```python
from build123d import *

# Parameters (mm, degrees)
SKETCH_1_W          = 80
SKETCH_1_H          = 118.5
SKETCH_1_W_2        = 35
SKETCH_1_H_2        = 15
EXTRUDE_1_DEPTH     = 3
CUT_EXTRUDE_2_REACH = 145.008
SKETCH_3_R          = 1.55
CUT_EXTRUDE_3_REACH = 145.008
SKETCH_4_R          = 1.55


with BuildPart() as part:
    # 草图1 → 凸台-拉伸1 (new body)
    with BuildSketch(Plane.XY):
        with Locations((40, 59.25)):
            Rectangle(SKETCH_1_W, SKETCH_1_H)
        with Locations((40, 59.25)):
            Rectangle(SKETCH_1_W_2, SKETCH_1_H_2, mode=Mode.SUBTRACT)
    extrude(amount=EXTRUDE_1_DEPTH)

    # 草图3 → 切除-拉伸2 (cut, up to next)
    with BuildSketch(Plane.XY.offset(3), mode=Mode.PRIVATE) as cut_extrude_2_sk1:
        with Locations((10, 113.5)):
            Circle(SKETCH_3_R)
    cut_extrude_2_tool1 = extrude(cut_extrude_2_sk1.sketch, amount=-CUT_EXTRUDE_2_REACH, mode=Mode.PRIVATE) & part.part
    # 草图3 → 切除-拉伸2 (cut, up to next)
    with BuildSketch(Plane.XY.offset(3), mode=Mode.PRIVATE) as cut_extrude_2_sk2:
        with Locations((70, 113.5)):
            Circle(SKETCH_3_R)
    cut_extrude_2_tool2 = extrude(cut_extrude_2_sk2.sketch, amount=-CUT_EXTRUDE_2_REACH, mode=Mode.PRIVATE) & part.part
    # 草图3 → 切除-拉伸2 (cut, up to next)
    with BuildSketch(Plane.XY.offset(3), mode=Mode.PRIVATE) as cut_extrude_2_sk3:
        with Locations((70, 5)):
            Circle(SKETCH_3_R)
    cut_extrude_2_tool3 = extrude(cut_extrude_2_sk3.sketch, amount=-CUT_EXTRUDE_2_REACH, mode=Mode.PRIVATE) & part.part
    # 草图3 → 切除-拉伸2 (cut, up to next)
    with BuildSketch(Plane.XY.offset(3), mode=Mode.PRIVATE) as cut_extrude_2_sk4:
        with Locations((10, 5)):
            Circle(SKETCH_3_R)
    cut_extrude_2_tool4 = extrude(cut_extrude_2_sk4.sketch, amount=-CUT_EXTRUDE_2_REACH, mode=Mode.PRIVATE) & part.part
    add(cut_extrude_2_tool1.solids().sort_by_distance((10, 113.5, 3))[0], mode=Mode.SUBTRACT)
    add(cut_extrude_2_tool2.solids().sort_by_distance((70, 113.5, 3))[0], mode=Mode.SUBTRACT)
    add(cut_extrude_2_tool3.solids().sort_by_distance((70, 5, 3))[0], mode=Mode.SUBTRACT)
    add(cut_extrude_2_tool4.solids().sort_by_distance((10, 5, 3))[0], mode=Mode.SUBTRACT)

    # 草图4 → 切除-拉伸3 (cut, up to next)
    with BuildSketch(Plane(origin=(0, 0, 0), x_dir=(-1, 0, 0), z_dir=(0, 0, -1)), mode=Mode.PRIVATE) as cut_extrude_3_sk1:
        with Locations((-67, 59.25)):
            Circle(SKETCH_4_R)
    cut_extrude_3_tool1 = extrude(cut_extrude_3_sk1.sketch, amount=-CUT_EXTRUDE_3_REACH, mode=Mode.PRIVATE) & part.part
    # 草图4 → 切除-拉伸3 (cut, up to next)
    with BuildSketch(Plane(origin=(0, 0, 0), x_dir=(-1, 0, 0), z_dir=(0, 0, -1)), mode=Mode.PRIVATE) as cut_extrude_3_sk2:
        with Locations((-13, 59.25)):
            Circle(SKETCH_4_R)
    cut_extrude_3_tool2 = extrude(cut_extrude_3_sk2.sketch, amount=-CUT_EXTRUDE_3_REACH, mode=Mode.PRIVATE) & part.part
    add(cut_extrude_3_tool1.solids().sort_by_distance((67, 59.25, 0))[0], mode=Mode.SUBTRACT)
    add(cut_extrude_3_tool2.solids().sort_by_distance((13, 59.25, 0))[0], mode=Mode.SUBTRACT)


solid = part.part
```
CAD build for the part. Positions are in the model's coordinates, mm. A direction names the side the tool comes from. Round coordinates to 2 decimals unless told otherwise and drop trailing zeros. Write each loop counter-clockwise with the first axis right and the second up, starting at its lowest first coordinate (ties: lowest second). Pieces come first, ordered by that corner, then holes. Notation, with made-up numbers: (20, -9.75) - (50, -9.75) arc R21 cw to (50, -2.75) - close; hole circle Ø2 at (65, -13). An arc over 180 degrees is marked (long way). Write item = value, one per line. Start each with the question number.
Q1. Mould opens along X. For faces 3 (the flat face through (80, 58, 1)), 4 (the flat face through (40, 66.75, 1)), 5 (the flat face through (0, 58, 1)) say: pulls with the +X half, pulls with the -X half, needs draft (parallel to the pull), parting line crosses it, or undercut.
Q2. Band-saw the part on D-D (x = 13). Give the cut face in (y, z).
Q3. Band-saw the part on B-B (z = 1.8). Give the cut face in (x, y).
Q4. Which spindle directions (+Z, -Z, +X, -X, +Y, -Y) get a long thin tool onto all of the face, cutting with end or side? Do faces 1 (the flat face through (39, 0, 1)), 2 (the flat face through (57.5, 59, 1)). Say none if no direction does.
Q5. Band-saw the part on C-C (x = 70). Give the cut face in (y, z).
Q6. Probe L1, parallel to Y at x = 70, z = 0.65; L2, parallel to Y at x = 13, z = 2.15; L3, parallel to Y at x = 27.5, z = 2. List the from-to ranges inside material, lowest first. Write a range as from..to.
Q7. Band-saw the part on A-A (x = 47). Give the cut face in (y, z).
Answers below:
q1.face_3 = pulls with the +X half
q1.face_4 = undercut
q1.face_5 = pulls with the -X half
q2.outline = (0, 0) - (57.7, 0) - (57.7, 3) - (0, 3) - close; (60.8, 0) - (118.5, 0) - (118.5, 3) - (60.8, 3) - close
q3.outline = (0, 0) - (80, 0) - (80, 118.5) - (0, 118.5) - close; hole circle Ø3.1 at (10, 5); hole circle Ø3.1 at (10, 113.5); hole circle Ø3.1 at (13, 59.25); hole (22.5, 51.75) - (57.5, 51.75) - (57.5, 66.75) - (22.5, 66.75) - close; hole circle Ø3.1 at (67, 59.25); hole circle Ø3.1 at (70, 5); hole circle Ø3.1 at (70, 113.5)
q4.face_1 = +Z, -Z, +X, -X, -Y
q4.face_2 = +Z, -Z
q5.outline = (0, 0) - (3.45, 0) - (3.45, 3) - (0, 3) - close; (6.55, 0) - (111.95, 0) - (111.95, 3) - (6.55, 3) - close; (115.05, 0) - (118.5, 0) - (118.5, 3) - (115.05, 3) - close
q6.L1 = 0..3.45, 6.55..111.95, 115.05..118.5
q6.L2 = 0..57.7, 60.8..118.5
q6.L3 = 0..51.75, 66.75..118.5
q7.outline = (0, 0) - (51.75, 0) - (51.75, 3) - (0, 3) - close; (66.75, 0) - (118.5, 0) - (118.5, 3) - (66.75, 3) - close
